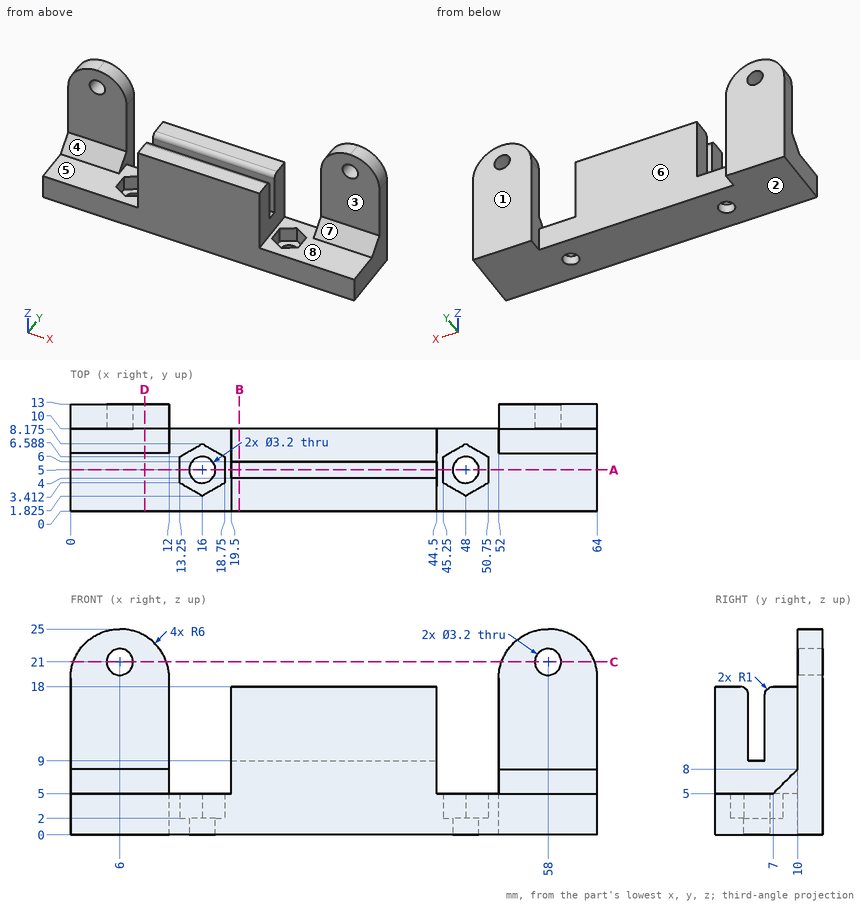
For this review, use the dimensioned drawing (mm, ordinates from the lowest corner) and the shaded views. A direction names the side the tool comes from. Coordinates: 2 decimals unless noted, no trailing zeros. Loops run counter-clockwise (first coordinate to the right, second up) from the corner with the lowest first, then second, coordinate; pieces in that order, holes last.
1. For line 1 (X direction, y = 6.5, z = 2.75); line 2 (Y direction, x = 16, z = 0.95); line 3 (Y direction, x = 16, z = 2.75) (1 decimal), list the stretches that pass through material, from the lowest coordinate up.
2. Add section D-D, the plane x = 9. Give the boundary of the cut face in (y, z).
3. Add section B-B, the plane x = 20.5. Give the boundary of the cut face in (y, z), then the cut area to 3 significant figures.
4. Add section A-A, the plane y = 5. Give the boundary of the cut face in (x, z).
5. Insertion check: P1, Ø1, axis at y = 6.5, z = 11.5, coming from the +X side; P2, Ø5, axis at x = 44.5, z = 11.5, coming from the +Y side; P3, Ø0.6, axis at x = 33.5, y = 5.5, coming from the +Z side. Each pin has a flat end and moves straight along its axis. Give the tip position at first contact, or say it passes through.
6. For the marked faces 1, 2, 3, 4 and 5, list the 3-axis set-ups (+Z, -Z, +X, -X, +Y, -Y) from which the entire face can be reached by the end or side of a thin tool; tool diameter is ignored.
7. Add section C-C, the plane z = 21. Give the boundary of the cut face in (x, y).
8. Mouldability with a two-part tool opening along X and no side actions: class the marked faces 6, 7 and 8 as +X half, -X half, draft (parallel to the pull), parting line (faces both ways), or undercut.
Result:
1. line 1: x = 0 to 13.25, 18.75 to 45.25, 50.75 to 64
1. line 2: y = 0 to 3.4, 6.6 to 10
1. line 3: y = 0 to 1.8, 8.2 to 10
2. outline: (0, 0) - (13, 0) - (13, 24.2) - (10, 24.2) - (10, 8) - (7, 5) - (0, 5) - close
3. outline: (0, 0) - (10, 0) - (10, 18) - (7, 18) arc R1 ccw to (6, 17) - (6, 9) - (4, 9) - (4, 17) arc R1 ccw to (3, 18) - (0, 18) - close
3. area: 162 mm2
4. outline: (0, 0) - (14.4, 0) - (14.4, 2) - (13.25, 2) - (13.25, 5) - (0, 5) - close; (17.6, 0) - (46.4, 0) - (46.4, 2) - (45.25, 2) - (45.25, 5) - (44.5, 5) - (44.5, 9) - (19.5, 9) - (19.5, 5) - (18.75, 5) - (18.75, 2) - (17.6, 2) - close; (49.6, 0) - (64, 0) - (64, 5) - (50.75, 5) - (50.75, 2) - (49.6, 2) - close
5. P1: stops at x = 44.5
5. P2: stops at y = 10
5. P3: stops at z = 9
6. face 1: +Z, -Z, +X, -X, +Y
6. face 2: -Z, +X, -X, +Y, -Y
6. face 3: +Z, +X, -Y
6. face 4: +Z, -X, -Y
6. face 5: +Z, -Y
7. outline: (0.34, 10) - (4.4, 10) - (4.4, 13) - (0.34, 13) - close; (7.6, 10) - (11.66, 10) - (11.66, 13) - (7.6, 13) - close; (52.34, 10) - (56.4, 10) - (56.4, 13) - (52.34, 13) - close; (59.6, 10) - (63.66, 10) - (63.66, 13) - (59.6, 13) - close
8. face 6: undercut
8. face 7: draft
8. face 8: undercut
